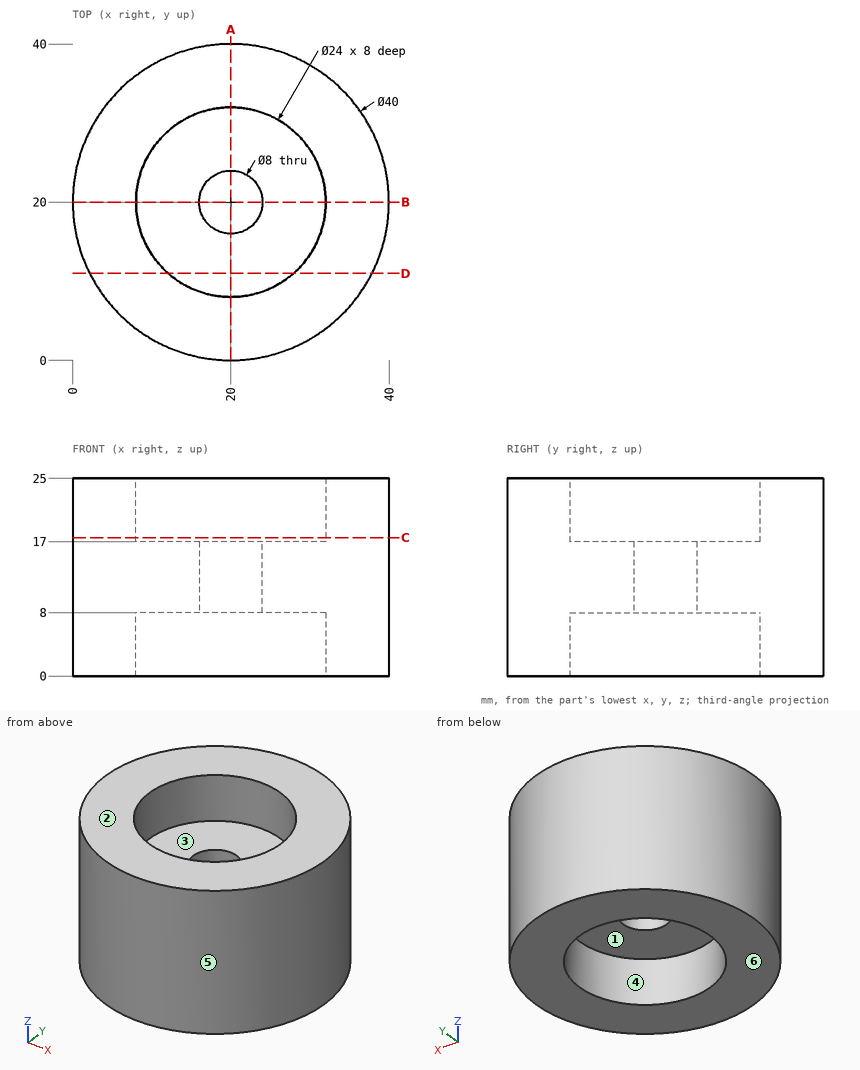
Can you work these out from the drawing? Everything is in mm from the part's minimum corner. A direction names the side the tool comes from. Give positions to 0.01 mm unless a question says otherwise; leave off trailing zeros. Order: outer loops, then holes, each group sorted by start corner. A loop starts at its lowest first (then second) coordinate and runs counter-clockwise, first axis right, second up.
Item 1: If we mould it in two halves opening along Y, with no side actions, what happens to the marked faces 4, 5 and 6? For each: pulls with the +Y half, pulls with the -Y half, needs draft (parallel to the pull), parting line crosses it, or undercut.
Item 2: For the marked faces 1, 2 and 3, which set-ups out of +Z, -Z, +X, -X, +Y, -Y let a thin tool reach every point of the face, with its end or its side?
Item 3: I need wall thicknesses on line 1 (Y direction, x = 20, z = 20.75); line 2 (Y direction, x = 20, z = 14.25); line 3 (Z direction, x = 19, y = 11.5). Which ranges of each line are inside material? Lowest first, please.
Item 4: I'm going to push flat-ended pins straight in: pin 1 (4 mm diameter, centred on y = 15, z = 5.5, fed in from -X); pin 2 (21.5 mm diameter, centred on x = 20, y = 20, fed in from +Z); pin 3 (3 mm diameter, centred on y = 9.5, z = 13.5, fed in from +X). Where does each tip first touch, or does it pass through?
Item 5: If we section it at C-C, the plane z = 17.5: Write out the boundary of the cut face in (x, y).
Item 6: If we section it at D-D, the plane y = 11: Write out the boundary of the cut face in (x, z).
Item 7: If we section it at A-A, the plane x = 20: Write out the boundary of the cut face in (y, z).
Values:
1. face 4: undercut
1. face 5: parting line crosses it
1. face 6: needs draft
2. face 1: -Z
2. face 2: +Z, +X, -X, +Y, -Y
2. face 3: +Z
3. line 1: y = 0 to 8, 32 to 40
3. line 2: y = 0 to 16, 24 to 40
3. line 3: z = 8 to 17
4. pin 1: stops at x = 0.23
4. pin 2: stops at z = 17
4. pin 3: stops at x = 37.86
5. outline: circle Ø40 at (20, 20); hole circle Ø24 at (20, 20)
6. outline: (2.14, 0) - (12.06, 0) - (12.06, 8) - (27.94, 8) - (27.94, 0) - (37.86, 0) - (37.86, 25) - (27.94, 25) - (27.94, 17) - (12.06, 17) - (12.06, 25) - (2.14, 25) - close
7. outline: (0, 0) - (8, 0) - (8, 8) - (16, 8) - (16, 17) - (8, 17) - (8, 25) - (0, 25) - close; (24, 8) - (32, 8) - (32, 0) - (40, 0) - (40, 25) - (32, 25) - (32, 17) - (24, 17) - close
